Verification items for the finished model (mm, model axes). A direction names the side the tool comes from. Give positions to 0.01 mm unless a question says otherwise; leave off trailing zeros. Write each loop counter-clockwise with the first axis right and the second up, starting at its lowest first coordinate (ties: lowest second). Pieces come first, ordered by that corner, then holes. Notation, with made-up numbers: (70.25, 9) -> (99.25, 9) arc R35 cw to (99.25, 47) -> close; hole circle Ø8 at (61.25, 84.25). An arc over 180 degrees is marked (long way). Write item = value, one per line.
from build123d import *

# Parameters (mm, degrees)
SKETCH_1_W          = 35
SKETCH_1_H          = 25
EXTRUDE_1_DEPTH     = 3
SKETCH_2_W          = 20
SKETCH_2_H          = 15
EXTRUDE_2_DEPTH     = 70
CUT_EXTRUDE_1_REACH = 78.102
SKETCH_3_W          = 15
SKETCH_3_H          = 11
CUT_EXTRUDE_2_REACH = 79.687
SKETCH_4_W          = 4
SKETCH_4_H          = 40
CUT_EXTRUDE_3_REACH = 75.229
SKETCH_5_R          = 1.5


with BuildPart() as part:
    # 草图1 → 凸台-拉伸1 (new body)
    with BuildSketch(Plane(origin=(0, 0, 0), x_dir=(1, 0, 0), z_dir=(0, 1, 0))):
        Rectangle(SKETCH_1_W, SKETCH_1_H)
    extrude(amount=EXTRUDE_1_DEPTH)

    # 草图2 → 凸台-拉伸2 (add)
    with BuildSketch(Plane(origin=(0, 3, 0), x_dir=(1, 0, 0), z_dir=(0, 1, 0))):
        Rectangle(SKETCH_2_W, SKETCH_2_H)
    extrude(amount=EXTRUDE_2_DEPTH)

    # 草图3 → 切除-拉伸1 (cut, up to next)
    with BuildSketch(Plane(origin=(0, 73, 0), x_dir=(1, 0, 0), z_dir=(0, 1, 0)), mode=Mode.PRIVATE) as cut_extrude_1_sk1:
        Rectangle(SKETCH_3_W, SKETCH_3_H)
    cut_extrude_1_tool1 = extrude(cut_extrude_1_sk1.sketch, amount=-CUT_EXTRUDE_1_REACH, mode=Mode.PRIVATE) & part.part
    add(cut_extrude_1_tool1.solids().sort_by_distance((0, 73, 0))[0], mode=Mode.SUBTRACT)

    # 草图4 → 切除-拉伸2 (cut, up to next)
    with BuildSketch(Plane.XY.offset(7.5), mode=Mode.PRIVATE) as cut_extrude_2_sk1:
        with Locations((-8, 38)):
            Rectangle(SKETCH_4_W, SKETCH_4_H)
    cut_extrude_2_tool1 = extrude(cut_extrude_2_sk1.sketch, amount=-CUT_EXTRUDE_2_REACH, mode=Mode.PRIVATE) & part.part
    add(cut_extrude_2_tool1.solids().sort_by_distance((-8, 38, 7.5))[0], mode=Mode.SUBTRACT)

    # 草图5 → 切除-拉伸3 (cut, up to next)
    with BuildSketch(Plane(origin=(0, 3, 0), x_dir=(1, 0, 0), z_dir=(0, 1, 0)), mode=Mode.PRIVATE) as cut_extrude_3_sk1:
        with Locations(Location((-14.5, 9.5, 0), (0, 0, 270))):
            Circle(SKETCH_5_R)
    cut_extrude_3_tool1 = extrude(cut_extrude_3_sk1.sketch, amount=-CUT_EXTRUDE_3_REACH, mode=Mode.PRIVATE) & part.part
    # 草图5 → 切除-拉伸3 (cut, up to next)
    with BuildSketch(Plane(origin=(0, 3, 0), x_dir=(1, 0, 0), z_dir=(0, 1, 0)), mode=Mode.PRIVATE) as cut_extrude_3_sk2:
        with Locations(Location((14.5, 9.5, 0), (0, 0, 270))):
            Circle(SKETCH_5_R)
    cut_extrude_3_tool2 = extrude(cut_extrude_3_sk2.sketch, amount=-CUT_EXTRUDE_3_REACH, mode=Mode.PRIVATE) & part.part
    # 草图5 → 切除-拉伸3 (cut, up to next)
    with BuildSketch(Plane(origin=(0, 3, 0), x_dir=(1, 0, 0), z_dir=(0, 1, 0)), mode=Mode.PRIVATE) as cut_extrude_3_sk3:
        with Locations(Location((-14.5, -9.5, 0), (0, 0, 270))):
            Circle(SKETCH_5_R)
    cut_extrude_3_tool3 = extrude(cut_extrude_3_sk3.sketch, amount=-CUT_EXTRUDE_3_REACH, mode=Mode.PRIVATE) & part.part
    # 草图5 → 切除-拉伸3 (cut, up to next)
    with BuildSketch(Plane(origin=(0, 3, 0), x_dir=(1, 0, 0), z_dir=(0, 1, 0)), mode=Mode.PRIVATE) as cut_extrude_3_sk4:
        with Locations(Location((14.5, -9.5, 0), (0, 0, 270))):
            Circle(SKETCH_5_R)
    cut_extrude_3_tool4 = extrude(cut_extrude_3_sk4.sketch, amount=-CUT_EXTRUDE_3_REACH, mode=Mode.PRIVATE) & part.part
    add(cut_extrude_3_tool1.solids().sort_by_distance((-14.5, 3, -9.5))[0], mode=Mode.SUBTRACT)
    add(cut_extrude_3_tool2.solids().sort_by_distance((14.5, 3, -9.5))[0], mode=Mode.SUBTRACT)
    add(cut_extrude_3_tool3.solids().sort_by_distance((-14.5, 3, 9.5))[0], mode=Mode.SUBTRACT)
    add(cut_extrude_3_tool4.solids().sort_by_distance((14.5, 3, 9.5))[0], mode=Mode.SUBTRACT)


solid = part.part
Item 1: Set-up check for faces 1 (the flat face through (0, 37, 5.5)), 2 (the flat face through (-10, 10, 0)), 3 (the flat face through (-8, 58, 0)), 4 (the flat face through (0, 38, -7.5)): record each of +Z, -Z, +X, -X, +Y, -Y from which the full face is reachable in a straight line by a thin tool's end or side.
Response values:
face_1 = +Y, -Y
face_2 = +Z, -Z, -X, +Y
face_3 = +Z, -Z, -X
face_4 = -Z, +X, -X, +Y
Item 2: Sectioned sample at A-A on z = -9.5. Record the cut outline in (x, y), then the cut area to 3 significant figures.
Response values:
outline = (-17.5, 0) -> (-16, 0) -> (-16, 3) -> (-17.5, 3) -> close; (-13, 0) -> (13, 0) -> (13, 3) -> (-13, 3) -> close; (16, 0) -> (17.5, 0) -> (17.5, 3) -> (16, 3) -> close
area = 87.0 mm^2
Item 3: Material ranges on line 1 (X direction, y = 1.05, z = 9.5); line 2 (X direction, y = 59, z = -2.5); line 3 (Z direction, x = -6.5, y = 13.5), recorded low to high.
Response values:
line_1 = -17.5 to -16, -13 to 13, 16 to 17.5
line_2 = -10 to -7.5, 7.5 to 10
line_3 = -7.5 to -5.5, 5.5 to 7.5
Item 4: Go/stop test with flat-tipped pins: P1, Ø4.5, axis at y = 66.5, z = -2.5, coming from the -X side; P2, Ø0.6, axis at y = 37.5, z = 7, coming from the -X side; P3, Ø5.5, axis at y = 64.5, z = 1, coming from the +X side. Record where each tip stops, or that it passes through.
Response values:
P1 = -10
P2 = -6
P3 = 10
Item 5: Sectioned sample at C-C on x = 5. Record the cut outline in (y, z), then the cut area to 3 significant figures.
Response values:
outline = (0, -12.5) -> (3, -12.5) -> (3, -7.5) -> (73, -7.5) -> (73, -5.5) -> (0, -5.5) -> close; (0, 5.5) -> (73, 5.5) -> (73, 7.5) -> (3, 7.5) -> (3, 12.5) -> (0, 12.5) -> close
area = 322 mm^2
Item 6: Sectioned sample at B-B on y = 17. Record the cut outline in (x, z), then the cut area to 3 significant figures.
Response values:
outline = (-10, -7.5) -> (10, -7.5) -> (10, 7.5) -> (-10, 7.5) -> close; hole (-7.5, -5.5) -> (7.5, -5.5) -> (7.5, 5.5) -> (-7.5, 5.5) -> close
area = 135 mm^2
Item 7: Sectioned sample at D-D on x = 14.5. Record the cut outline in (y, z).
Response values:
outline = (0, -12.5) -> (3, -12.5) -> (3, -11) -> (0, -11) -> close; (0, -8) -> (3, -8) -> (3, 8) -> (0, 8) -> close; (0, 11) -> (3, 11) -> (3, 12.5) -> (0, 12.5) -> close
Item 8: Mould release check, pull along X, two halves, no side actions. Record for faces 5 (the flat face through (-8, 18, 0)), 6 (the flat face through (-6, 38, -6)), 7 (the cylindrical face through (-14.43, 1.52, 8)): +X half, -X half, draft (parallel to the pull), parting line (faces both ways), or undercut.
Response values:
face_5 = draft
face_6 = -X half
face_7 = undercut
